```python
from build123d import *

# Parameters (mm, degrees)
SKETCH2_R                 = 41.27500000000001
SKETCH2_R_2               = 34.925000000000004
BOSS_EXTRUDE1_DEPTH       = 3.555999999999654
SKETCH54_R                = 41.27500000000001
SKETCH54_R_2              = 34.92500000000001
BOSS_EXTRUDE2_DEPTH       = 25.4
BOSS_EXTRUDE2_TAPER       = 10.000000000000021
BOSS_EXTRUDE3_START       = -18.006319777
BOSS_EXTRUDE3_OUTLINE_R   = 38.1
BOSS_EXTRUDE3_DEPTH       = 3.81
BOSS_EXTRUDE5_REACH       = 72.778
SKETCH63_R                = 3.175000000000002
SKETCH63_R_2              = 3.175000000000009
SKETCH63_R_3              = 3.1750000000000047
SKETCH63_R_4              = 3.1750000000000056
F_3_0MM_DOWEL_HOLE4_D     = 2.85
F_3_0MM_DOWEL_HOLE4_DEPTH = 6.858
F_3_0MM_DOWEL_HOLE3_D     = 2.9
CUT_EXTRUDE2_REACH        = 126.878
SKETCH58_W                = 12.700000000000001
SKETCH58_H                = 21.266668123278706
SKETCH60_R                = 1.4249999999999978
SKETCH60_R_2              = 1.4250000000000005
CUT_EXTRUDE4_DEPTH        = 70.71188168256496
SKETCH64_R                = 1.425000000000001
SKETCH64_R_2              = 1.4249999999999978
SKETCH64_R_3              = 1.4499999999999962
BOSS_EXTRUDE6_DEPTH       = 2.54
CHAMFER1_SIZE             = 7.62


with BuildPart() as part:
    # Sketch2 → Boss-Extrude1 (new body)
    with BuildSketch(Plane(origin=(0, 0.7215916123591171, 0), x_dir=(1, 0, 0), z_dir=(0, 0, 1))):
        with Locations((11.43, -1.4797279014976155)):
            Circle(SKETCH2_R)
        with Locations((11.43, -1.4797279014976155)):
            Circle(SKETCH2_R_2, mode=Mode.SUBTRACT)
    extrude(amount=BOSS_EXTRUDE1_DEPTH)

    # Sketch54 → Boss-Extrude2 (add)
    with BuildSketch(Plane(origin=(0, 0, 0), x_dir=(-1, 0, 0), z_dir=(0, 0, -1))):
        with Locations((-11.43, -0.7581362891384984)):
            Circle(SKETCH54_R)
        with Locations(Location((-11.43, -0.7581362891384984, 0), (0, 0, 180))):
            Circle(SKETCH54_R_2, mode=Mode.SUBTRACT)
    extrude(amount=BOSS_EXTRUDE2_DEPTH, taper=BOSS_EXTRUDE2_TAPER)

    # Boss-Extrude3: read off the stored shape, not the designer's step
    # Boss-Extrude3 outline → Boss-Extrude3 (add)
    with BuildSketch(Plane.XY.offset(BOSS_EXTRUDE3_START)):
        with Locations((11.43, -0.758136289)):
            Circle(BOSS_EXTRUDE3_OUTLINE_R)
    extrude(amount=BOSS_EXTRUDE3_DEPTH)

    # Sketch63 → Boss-Extrude5 (add, up to next)
    with BuildSketch(Plane.XY.offset(3.555999999999654), mode=Mode.PRIVATE) as boss_extrude5_sk1:
        with Locations((-7.620000000000007, 18.2918637108615)):
            Circle(SKETCH63_R)
    boss_extrude5_tool1 = extrude(boss_extrude5_sk1.sketch, amount=-BOSS_EXTRUDE5_REACH, mode=Mode.PRIVATE) - part.part
    # Sketch63 → Boss-Extrude5 (add, up to next)
    with BuildSketch(Plane.XY.offset(3.555999999999654), mode=Mode.PRIVATE) as boss_extrude5_sk2:
        with Locations((30.479999999999997, 18.291863710861506)):
            Circle(SKETCH63_R_2)
    boss_extrude5_tool2 = extrude(boss_extrude5_sk2.sketch, amount=-BOSS_EXTRUDE5_REACH, mode=Mode.PRIVATE) - part.part
    # Sketch63 → Boss-Extrude5 (add, up to next)
    with BuildSketch(Plane.XY.offset(3.555999999999654), mode=Mode.PRIVATE) as boss_extrude5_sk3:
        with Locations((30.48, -19.8081362891385)):
            Circle(SKETCH63_R_3)
    boss_extrude5_tool3 = extrude(boss_extrude5_sk3.sketch, amount=-BOSS_EXTRUDE5_REACH, mode=Mode.PRIVATE) - part.part
    # Sketch63 → Boss-Extrude5 (add, up to next)
    with BuildSketch(Plane.XY.offset(3.555999999999654), mode=Mode.PRIVATE) as boss_extrude5_sk4:
        with Locations((-7.620000000000007, -19.8081362891385)):
            Circle(SKETCH63_R_4)
    boss_extrude5_tool4 = extrude(boss_extrude5_sk4.sketch, amount=-BOSS_EXTRUDE5_REACH, mode=Mode.PRIVATE) - part.part
    add(boss_extrude5_tool1.solids().sort_by_distance((-7.62, 18.291864, 3.556))[0])
    add(boss_extrude5_tool2.solids().sort_by_distance((30.48, 18.291864, 3.556))[0])
    add(boss_extrude5_tool3.solids().sort_by_distance((30.48, -19.808136, 3.556))[0])
    add(boss_extrude5_tool4.solids().sort_by_distance((-7.62, -19.808136, 3.556))[0])

    # Ø3.0mm Dowel Hole4
    with Locations(Plane.XY.offset(3.555999999999654)):
        with Locations((-7.62, 18.291863711), (30.48, 18.291863711), (30.48, -19.808136289), (-7.62, -19.808136289)):
            Hole(F_3_0MM_DOWEL_HOLE4_D / 2, depth=F_3_0MM_DOWEL_HOLE4_DEPTH)

    # Ø3.0mm Dowel Hole3 (through all)
    with Locations(Plane(origin=(0, 0, -18.006319777286198), x_dir=(-1, 0, 0), z_dir=(0, 0, -1))):
        with Locations((-11.43, -0.758136289)):
            Hole(F_3_0MM_DOWEL_HOLE3_D / 2)

    # Cut-Extrude2: up to this cone (the profile starts outside it)
    cut_extrude2_end = Plane(origin=(11.43, -0.7581362891384984, -11.65632), z_dir=(0, 0, -1)) * Cone(7.999516737370435, 65.961130686173, 328.7166474235434, mode=Mode.PRIVATE)
    # Sketch58 → Cut-Extrude2 (cut, up to the surface)
    with BuildSketch(Plane(origin=(-63.5, 0, 0), x_dir=(0, 0, -1), z_dir=(1, 0, 0)), mode=Mode.PRIVATE) as cut_extrude2_sk1:
        with Locations((11.656319777286228, -0.08753137128510957)):
            Rectangle(SKETCH58_W, SKETCH58_H)
    cut_extrude2_tool1 = extrude(cut_extrude2_sk1.sketch, amount=CUT_EXTRUDE2_REACH, mode=Mode.PRIVATE) - cut_extrude2_end
    add(cut_extrude2_tool1.solids().sort_by_distance((-63.5, -0.087531, -11.65632))[0], mode=Mode.SUBTRACT)

    # Sketch60 → Cut-Extrude4 (cut, through all)
    with BuildSketch(Plane.XY.offset(-14.196319777286197)):
        with Locations((18.43, -0.7581362891384957)):
            Circle(SKETCH60_R)
        with Locations((4.429999999999999, -0.7581362891384984)):
            Circle(SKETCH60_R_2)
    extrude(amount=-CUT_EXTRUDE4_DEPTH, mode=Mode.SUBTRACT)

    # Sketch64 → Boss-Extrude6 (add)
    with BuildSketch(Plane(origin=(0, 0, -18.006319777286198), x_dir=(-1, 0, 0), z_dir=(0, 0, -1))):
        with BuildLine():
            ThreePointArc((25.344366452837203, -10.720865432924475), (26.663599038852283, -0.05977229582778121), (24.954487952256596, 10.545802690354252))
            ThreePointArc((24.954487952256596, 10.545802690354252), (-49.52359903885228, -1.4565002824492193), (25.344366452837203, -10.720865432924475))
        make_face()
        with Locations(Location((-4.429999999999999, -0.7581362891384984, 0), (0, 0, 180))):
            Circle(SKETCH64_R, mode=Mode.SUBTRACT)
        with Locations(Location((-18.43, -0.7581362891384957, 0), (0, 0, 180))):
            Circle(SKETCH64_R_2, mode=Mode.SUBTRACT)
        with Locations((-11.43, -0.7581362891384984)):
            Circle(SKETCH64_R_3, mode=Mode.SUBTRACT)
    extrude(amount=BOSS_EXTRUDE6_DEPTH)

    # Chamfer1
    # the kernel refuses this chamfer: 7.62 mm, written as the material it adds along each edge
    with BuildSketch(Plane(origin=(-7.620000000000007, 18.2918637108615, -14.196319777000001), x_dir=(1, 0, 0), z_dir=(0, -1, 0))) as chamfer1_piece_1:
        Polygon((3.1750000000000016 + CHAMFER1_SIZE, 0), (3.1750000000000016, CHAMFER1_SIZE), (3.1750000000000016, 0), align=None)
    revolve(axis=Axis((-7.620000000000007, 18.2918637108615, -14.196319777000001), (0, 0, 1)))
    with BuildSketch(Plane(origin=(30.479999999999997, 18.291863710861506, -14.196319777000001), x_dir=(1, 0, 0), z_dir=(0, -1, 0))) as chamfer1_piece_2:
        Polygon((3.1750000000000043 + CHAMFER1_SIZE, 0), (3.1750000000000043, CHAMFER1_SIZE), (3.1750000000000043, 0), align=None)
    revolve(axis=Axis((30.479999999999997, 18.291863710861506, -14.196319777000001), (0, 0, 1)))
    with BuildSketch(Plane(origin=(30.48, -19.8081362891385, -14.196319777000001), x_dir=(1, 0, 0), z_dir=(0, -1, 0))) as chamfer1_piece_3:
        Polygon((3.1750000000000007 + CHAMFER1_SIZE, 0), (3.1750000000000007, CHAMFER1_SIZE), (3.1750000000000007, 0), align=None)
    revolve(axis=Axis((30.48, -19.8081362891385, -14.196319777000001), (0, 0, 1)))
    with BuildSketch(Plane(origin=(-7.620000000000007, -19.8081362891385, -14.196319777000001), x_dir=(1, 0, 0), z_dir=(0, -1, 0))) as chamfer1_piece_4:
        Polygon((3.175000000000005 + CHAMFER1_SIZE, 0), (3.175000000000005, CHAMFER1_SIZE), (3.175000000000005, 0), align=None)
    revolve(axis=Axis((-7.620000000000007, -19.8081362891385, -14.196319777000001), (0, 0, 1)))


solid = part.part
```
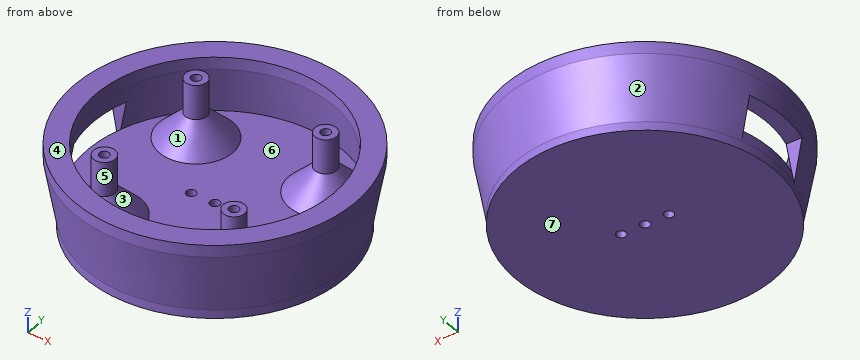
Check sheet for the modelled part. Datum: model origin and axes. Units: mm. Face numbers are marked on the shaded views. A direction names the side the tool comes from. Give positions to 0.01 mm unless a question says otherwise; leave off trailing zeros. Write each loop counter-clockwise with the first axis right and the second up, starting at its lowest first coordinate (ties: lowest second). Pieces come first, ordered by that corner, then holes. Notation, with made-up numbers: (86.25, 30.5) -> (106.25, 30.5) arc R24 cw to (106.25, 46.5) -> close; hole circle Ø10 at (25.25, -21.75). An arc over 180 degrees is marked (long way). Use CSV: the item, a comma, the result in double quotes. Start each with the question number.
Q1. Cross-section at A-A on x = 11.43. Enter the section's corners in (y, z).
Q2. Cross-section at C-C on z = -15.75. Enter the section's corners in (x, y) (3 decimals), and give its area (3 significant figures).
Q3. Scan lines: line 1 along X through (y, z) = (-19, -4); line 2 along Y through (x, z) = (-7.62, 1); line 3 along X through (y, z) = (14, -11). Record each from-to range of solid material in increasing order.
Q4. Release check for a two-part mould opening along X. For the marked faces 1, 2, 3 and 4 record: +X half, -X half, draft (parallel to the pull), parting line (faces both ways), or undercut.
Q5. Tool access check on the marked faces 5, 6 and 7. Record the directions out of +Z, -Z, +X, -X, +Y, -Y that give a thin tool (end or side, any length) a straight path to the whole face; none if there is none.
Q6. Depth check by flat-ended pin: P1, Ø12, axis at x = -12, y = -8, coming from the +Z side; P2, Ø1.4, axis at x = -25.5, z = -11, coming from the -Y side; P3, Ø2.5, axis at x = 30.48, y = 18.29, coming from the +Z side; P4, Ø1.7, axis at x = 18.43, y = -0.76, coming from the +Z side. Enter the tip coordinate at first touch or a pass-through.
Q7. Cross-section at B-B on z = -8.5. Enter the section's corners in (x, y), and give its area (3 significant figures).
Working result:
1,outline,"(-42.03, 0) -> (-38.86, -18.01) -> (-38.86, -20.55) -> (-2.21, -20.55) -> (-2.21, -14.2) -> (-38.19, -14.2) -> (-35.68, 0) -> (-35.68, 3.56) -> (-42.03, 3.56) -> close; (0.69, -20.55) -> (37.34, -20.55) -> (37.34, -18.01) -> (40.52, 0) -> (40.52, 3.56) -> (34.17, 3.56) -> (34.17, 0) -> (36.67, -14.2) -> (0.69, -14.2) -> close"
2,outline,"(-25.756, -10.721) arc R38.498 ccw (long way) to (-25.371, 10.546) -> (-24.538, 10.546) arc R37.702 ccw to (-24.932, -10.721) -> close; hole circle Ø2.85 at (4.43, -0.758); hole circle Ø2.9 at (11.43, -0.758); hole circle Ø2.85 at (18.43, -0.758)"
2,area,"4,620 mm^2"
3,line 1,"x = -24.81 to -19.18, -10.69 to -4.55, 27.41 to 33.55, 42.04 to 47.67"
3,line 2,"y = -37.37 to -30.03, -22.98 to -21.23, -18.38 to -16.63, 15.12 to 16.87, 19.72 to 21.47, 28.51 to 35.86"
3,line 3,"x = -25.03 to -22.35, -13.89 to -1.35, 24.21 to 36.75, 45.21 to 47.89"
4,face 1,"undercut"
4,face 2,"parting line"
4,face 3,"undercut"
4,face 4,"draft"
5,face 5,"+Z"
5,face 6,"none"
5,face 7,"-Z, +X, -X, +Y, -Y"
6,P1,"stops at z = -10"
6,P2,"stops at y = -16.11"
6,P3,"stops at z = -3.3"
6,P4,"passes through"
7,outline,"(-27.08, -10.72) arc R39.78 ccw (long way) to (-26.71, 10.55) -> (-23.2, 10.55) arc R36.42 cw (long way) to (-23.6, -10.72) -> close; circle Ø10.2 at (-7.62, -19.81); circle Ø10.2 at (-7.62, 18.29); circle Ø10.2 at (30.48, -19.81); circle Ø10.2 at (30.48, 18.29)"
7,area,"1,060 mm^2"
